from build123d import *

# Parameters (mm, degrees)
SKETCH1_W                 = 78
SKETCH1_H                 = 78
BOSS_EXTRUDE1_DEPTH       = 10
SHELL1_T                  = -3
SHELL1_THICKNESS_2_FACE_W = 72
SHELL1_THICKNESS_2_FACE_H = 72
SHELL1_THICKNESS_2_DEPTH  = 2
SKETCH10_R                = 1.25
CUT_EXTRUDE7_DEPTH        = 57.053545829
FILLET5_R                 = 2
FILLET6_R                 = 1
BOSS_EXTRUDE2_START       = 3
SKETCH15_W                = 6
SKETCH15_H                = 9
SKETCH15_R                = 1.25
BOSS_EXTRUDE2_DEPTH       = 3
FILLET7_R                 = 2
FILLET7_OF_MIRROR5_R      = 2
SKETCH16_R                = 1.75
CUT_EXTRUDE9_DEPTH        = 86.12343978
SKETCH20_W                = 19.5
SKETCH20_H                = 11
BOSS_EXTRUDE3_DEPTH       = 10
CUT_EXTRUDE10_START       = -1.5
SKETCH21_W                = 16
SKETCH21_H                = 9.5
CUT_EXTRUDE10_DEPTH       = 55.553545829
SKETCH22_W                = 12
SKETCH22_H                = 5.5
CUT_EXTRUDE11_DEPTH       = 56.805465682
SKETCH22_2_W              = 13
SKETCH22_2_H              = 6.5
SKETCH22_2_W_2            = 12
SKETCH22_2_H_2            = 5.5
EXTRUDE_THIN3_DEPTH       = 8.5
FILLET8_R                 = 2
SKETCH26_W                = 22.5
SKETCH26_H                = 6
BOSS_EXTRUDE4_DEPTH       = 3
SKETCH13_R                = 1.5
CUT_EXTRUDE8_DEPTH        = 57.053545829
SKETCH28_W                = 3
SKETCH28_H                = 61
SKETCH28_H_2              = 72
BOSS_EXTRUDE5_DEPTH       = 5
SKETCH29_W                = 72
SKETCH29_H                = 3
BOSS_EXTRUDE6_DEPTH       = 5
CHAMFER1_SIZE2            = 14.92820323
CHAMFER1_SIZE             = 4
CHAMFER2_SIZE             = 4


with BuildPart() as part:
    # Sketch1 → Boss-Extrude1 (new body)
    with BuildSketch(Plane.XY):
        Rectangle(SKETCH1_W, SKETCH1_H)
    extrude(amount=BOSS_EXTRUDE1_DEPTH)

    # Shell1
    shell1_openings = [part.faces().sort_by_distance(p)[0] for p in [
        (0, 0, 10),
    ]]
    offset(amount=SHELL1_T, openings=shell1_openings, kind=Kind.INTERSECTION)

    # Shell1 thickness 2 face (on inner face of the shell) → Shell1 thickness 2 (cut)
    with BuildSketch(Plane(origin=(0, 0, 3), x_dir=(-1, 0, 0), z_dir=(0, 0, -1))):
        Rectangle(SHELL1_THICKNESS_2_FACE_W, SHELL1_THICKNESS_2_FACE_H)
    extrude(amount=SHELL1_THICKNESS_2_DEPTH, mode=Mode.SUBTRACT)

    # Sketch10 → Cut-Extrude7 (cut, symmetric)
    with BuildSketch(Plane(origin=(0, 0, 0), x_dir=(1, 0, 0), z_dir=(0, 1, 0))):
        with Locations(Location((-30, -5, 0), (0, 0, 270))):
            Circle(SKETCH10_R)
    cut_extrude7 = extrude(amount=CUT_EXTRUDE7_DEPTH, both=True, mode=Mode.SUBTRACT)

    # Mirror4: Cut-Extrude7 across plane
    add(cut_extrude7.mirror(Plane(origin=(0, 0, 0), x_dir=(0, 0, 1), z_dir=(1, 0, 0))), mode=Mode.SUBTRACT)

    # Fillet5
    fillet5_edges = [part.edges().sort_by_distance(p)[0] for p in [
        (39, -39, 5),
        (-39, -39, 5),
        (-39, 39, 5),
        (39, 39, 5),
    ]]
    fillet(fillet5_edges, radius=FILLET5_R)

    # Fillet6
    fillet6_edges = [part.edges().sort_by_distance(p)[0] for p in [
        (36, -36, 5.5),
        (36, 36, 5.5),
        (-36, 36, 5.5),
        (-36, -36, 5.5),
    ]]
    fillet(fillet6_edges, radius=FILLET6_R)

    # Sketch15 → Boss-Extrude2 (add)
    with BuildSketch(Plane(origin=(0, -36, 0), x_dir=(1, 0, 0), z_dir=(0, 1, 0)).offset(BOSS_EXTRUDE2_START)):
        with Locations((-30, -5.5)):
            Rectangle(SKETCH15_W, SKETCH15_H)
        with Locations(Location((-30, -5, 0), (0, 0, 270))):
            Circle(SKETCH15_R, mode=Mode.SUBTRACT)
    boss_extrude2 = extrude(amount=-BOSS_EXTRUDE2_DEPTH)

    # Fillet7
    fillet7_edges = [part.edges().sort_by_distance(p)[0] for p in [
        (-33, -36, 5.5),
        (-27, -36, 5.5),
    ]]
    fillet(fillet7_edges, radius=FILLET7_R - 0.0001)  # a hair under: the kernel refuses the full size

    # Mirror5: Boss-Extrude2 across plane
    add(boss_extrude2.mirror(Plane(origin=(0, 0, 0), x_dir=(0, 0, 1), z_dir=(1, 0, 0))))

    # Fillet7 of Mirror5
    fillet7_of_mirror5_edges = [part.edges().sort_by_distance(p)[0] for p in [
        (33, -36, 5.5),
        (27, -36, 5.5),
    ]]
    fillet(fillet7_of_mirror5_edges, radius=FILLET7_OF_MIRROR5_R - 0.0001)  # a hair under: the kernel refuses the full size

    # Sketch16 → Cut-Extrude9 (cut, through all)
    with BuildSketch(Plane.XZ.offset(-36)):
        with Locations(Location((-30, 5, 0), (0, 0, 270))):
            Circle(SKETCH16_R)
        with Locations(Location((30, 5, 0), (0, 0, 270))):
            Circle(SKETCH16_R)
    extrude(amount=-CUT_EXTRUDE9_DEPTH, mode=Mode.SUBTRACT)

    # Sketch20 → Boss-Extrude3 (add)
    with BuildSketch(Plane(origin=(0, 0, 0), x_dir=(-1, 0, 0), z_dir=(0, 0, -1))):
        with Locations((17.25, -30.5)):
            Rectangle(SKETCH20_W, SKETCH20_H)
    extrude(amount=-BOSS_EXTRUDE3_DEPTH)

    # Sketch21 → Cut-Extrude10 (cut, through all)
    with BuildSketch(Plane.XY.offset(10).offset(CUT_EXTRUDE10_START)):
        with Locations((-17.25, -32)):
            Rectangle(SKETCH21_W, SKETCH21_H)
    extrude(amount=-CUT_EXTRUDE10_DEPTH, mode=Mode.SUBTRACT)

    # Sketch22 → Cut-Extrude11 (cut, through all)
    with BuildSketch(Plane(origin=(0, 0, 8.5), x_dir=(-1, 0, 0), z_dir=(0, 0, -1))):
        with Locations((17.25, -32)):
            Rectangle(SKETCH22_W, SKETCH22_H)
    extrude(amount=-CUT_EXTRUDE11_DEPTH, mode=Mode.SUBTRACT)

    # Sketch22<2> → Extrude-Thin3 (add)
    with BuildSketch(Plane(origin=(0, 0, 8.5), x_dir=(-1, 0, 0), z_dir=(0, 0, -1))):
        with Locations((17.25, -32)):
            Rectangle(SKETCH22_2_W, SKETCH22_2_H)
        with Locations((17.25, -32)):
            Rectangle(SKETCH22_2_W_2, SKETCH22_2_H_2, mode=Mode.SUBTRACT)
    extrude(amount=EXTRUDE_THIN3_DEPTH)

    # Fillet8
    fillet8_edges = [part.edges().sort_by_distance(p)[0] for p in [
        (-7.5, -25, 5.5),
        (-27, -25, 5.5),
    ]]
    fillet(fillet8_edges, radius=FILLET8_R)

    # Sketch26 → Boss-Extrude4 (add)
    with BuildSketch(Plane.XY.offset(1)):
        with Locations((3.75, -33)):
            Rectangle(SKETCH26_W, SKETCH26_H)
    extrude(amount=BOSS_EXTRUDE4_DEPTH)

    # Sketch13 → Cut-Extrude8 (cut, through all)
    with BuildSketch(Plane.XY):
        with Locations((0, -34)):
            Circle(SKETCH13_R)
    extrude(amount=CUT_EXTRUDE8_DEPTH, mode=Mode.SUBTRACT)

    # Sketch28 → Boss-Extrude5 (add)
    with BuildSketch(Plane.XY.offset(1)):
        with Locations((-16.5, 5.5)):
            Rectangle(SKETCH28_W, SKETCH28_H)
        with Locations((16.5, 0)):
            Rectangle(SKETCH28_W, SKETCH28_H_2)
    extrude(amount=BOSS_EXTRUDE5_DEPTH)

    # Sketch29 → Boss-Extrude6 (add)
    with BuildSketch(Plane.XY.offset(1)):
        Rectangle(SKETCH29_W, SKETCH29_H)
    extrude(amount=BOSS_EXTRUDE6_DEPTH)

    # Chamfer1
    chamfer1_edges = [part.edges().sort_by_distance(p)[0] for p in [
        (-16.5, -25, 6),
    ]]
    chamfer1_side = [part.faces().sort_by_distance(p)[0] for p in [
        (-16.5, -25, 6.08),
    ]]
    chamfer(chamfer1_edges, length=CHAMFER1_SIZE - 0.0001, length2=CHAMFER1_SIZE2 - 0.0001, reference=chamfer1_side[0])  # a hair under: the kernel refuses the full size

    # Chamfer2
    chamfer2_edges = [part.edges().sort_by_distance(p)[0] for p in [
        (-16.5, 36, 6),
        (16.5, -36, 6),
        (16.5, 36, 6),
        (36, 0, 6),
        (-36, 0, 6),
    ]]
    chamfer(chamfer2_edges, length=CHAMFER2_SIZE - 0.0001)  # a hair under: the kernel refuses the full size


solid = part.part
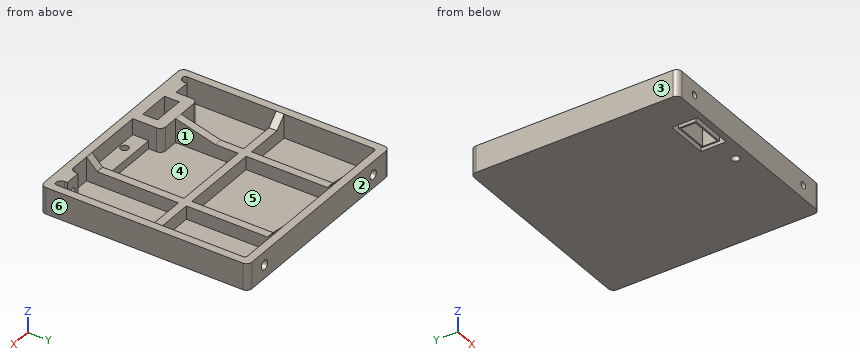
Could you check a few things on this model? Use its own coordinates, in mm. Face numbers are marked on the shaded views. A direction names the side the tool comes from. Coordinates: 2 decimals unless noted, no trailing zeros. Write each loop counter-clockwise with the first axis right and the second up, starting at its lowest first coordinate (ties: lowest second). Pieces come first, ordered by that corner, then holes. Notation, with made-up numbers: (38, -31) - (43, -31) arc R11 cw to (43, -15) - close; hole circle Ø10 at (67, -9). An arc over 180 degrees is marked (long way). Put each result on its own line as item: value. Start each with the question number.
Q1. I'm going to push flat-ended pins straight in: P1, Ø1.5, axis at x = -6.5, y = -28, coming from the -Z side; P2, Ø1, axis at x = 11.5, y = 22.5, coming from the +Z side. Where does each tip first touch, or does it pass through?
Q2. I want a section at A-A on x = -30. Write out the boundary of the cut face in (y, z), plus the area to 4 significant figures.
Q3. I want a section at B-B on x = 0. Write out the boundary of the cut face in (y, z).
Q4. Thinking about a two-plate mould opening in Y: for the marked faces 1, 2, 3 and 4, which applies, pulls with the +Y half, pulls with the -Y half, needs draft (parallel to the pull), parting line crosses it, or undercut?
Q5. Which directions (+Z, -Z, +X, -X, +Y, -Y) give clear straight access to the entire face, cutting with the end or side of a thin tool? Please do the marked faces 5 and 6.
Q6. Please list where these lines run through material, in increasing order: L1, parallel to X at y = 36.8, z = 5; L2, parallel to Y at x = -6.5, z = 3.5; L3, parallel to X at y = -22, z = 7.
Q7. I want a section at C-C on z = 5. Count the separate pieces of the cut face and the enclosed holes in it, plus the area to 3 significant figures.
Q8. I want a section at D-D on y = 22. Write out the boundary of the cut face in (x, z).
Checks:
1. P1: z = 0
1. P2: z = 1
2. outline: (-39, 0) - (39, 0) - (39, 3.25) - (36, 3.25) - (36, 1) - (1.5, 1) - (1.5, 6) - (-1.5, 6) - (-1.5, 1) - (-33, 1) - (-33, 3.75) - (-39, 3.75) - close; (-39, 6.25) - (-33, 6.25) - (-33, 10) - (-39, 10) - close; (36, 6.75) - (39, 6.75) - (39, 10) - (36, 10) - close
2. area: 148.5 mm²
3. outline: (-39, 0) - (-35.5, 0) - (-35.5, 4) - (-36, 4) - (-36, 10) - (-39, 10) - close; (-32.5, 0) - (39, 0) - (39, 10) - (36, 10) - (36, 1) - (1.5, 1) - (1.5, 6) - (-1.5, 6) - (-1.5, 1) - (-30, 1) - (-30, 4) - (-32.5, 4) - close
4. face 1: undercut
4. face 2: pulls with the +Y half
4. face 3: needs draft
4. face 4: undercut
5. face 5: +Z
5. face 6: +Z, -Z, +X, +Y, -Y
6. L1: -39 to -31.75, -28.25 to 28.25, 31.75 to 39
6. L2: -39 to -30, -1.5 to 1.5, 36 to 39
6. L3: -39 to -36, -18 to -15, 36 to 39
7. separate pieces: 2
7. enclosed holes: 4
7. area: 1,560 mm²
8. outline: (-39, 0) - (39, 0) - (39, 10) - (36, 10) - (36, 1) - (18, 1) - (18, 6) - (15, 6) - (15, 1) - (-15, 1) - (-15, 6) - (-18, 6) - (-18, 1) - (-36, 1) - (-36, 10) - (-39, 10) - close
